Design review of the part shown in the three views and the two pictorial views. Dimensions are in mm from the part's minimum x, y and z. A direction names the side the tool comes from. Coordinates: 2 decimals unless noted, no trailing zeros. Order: outer loops, then holes, each group sorted by start corner. A loop starts at its lowest first (then second) coordinate and runs counter-clockwise, first axis right, second up. Notation, with made-up numbers: (66.5, 69.5) -> (83.5, 69.5) arc R17 ccw to (83.5, 84.5) -> close; hole circle Ø11 at (47.25, 12). An arc over 180 degrees is marked (long way). Answer as a JSON object with one key per item and string values. Group by question number.
1) Wall thickness on L1, parallel to Z at x = 47, y = 11.5; L2, parallel to X at y = 7, z = 19.5; L3, parallel to Y at x = 14, z = 3: over which ranges is each line inside the solid? List them lowest first.
2) Add section A-A, the plane x = 25. Write out the cut boundary in (y, z), then the cut area to 3 significant figures.
3) Add section B-B, the plane y = 6.5. Write out the cut boundary in (x, z), then the cut area to 3 significant figures.
4) Add section D-D, the plane x = 10. Write out the cut boundary in (y, z).
5) For pin 1 (1.6 mm diameter, centred on x = 25.5, z = 38.5, fed in from -Y); pin 2 (13 mm diameter, centred on x = 29, y = 5.5, fed in from +Z); pin 3 (12 mm diameter, centred on x = 16.5, y = 17, fed in from -Z), all flat-tipped, find the tip position at first contact; note any pin that passes through.
6) Add section C-C, the plane z = 33.5. Write out the cut boundary in (x, y).
7) Machinability: for the marked faces 1, 2 and 3, which of the approach directions +Z, -Z, +X, -X, +Y, -Y give a long, thin tool a straight path to every point of the face, cutting with its end or side? Answer none if there is none.
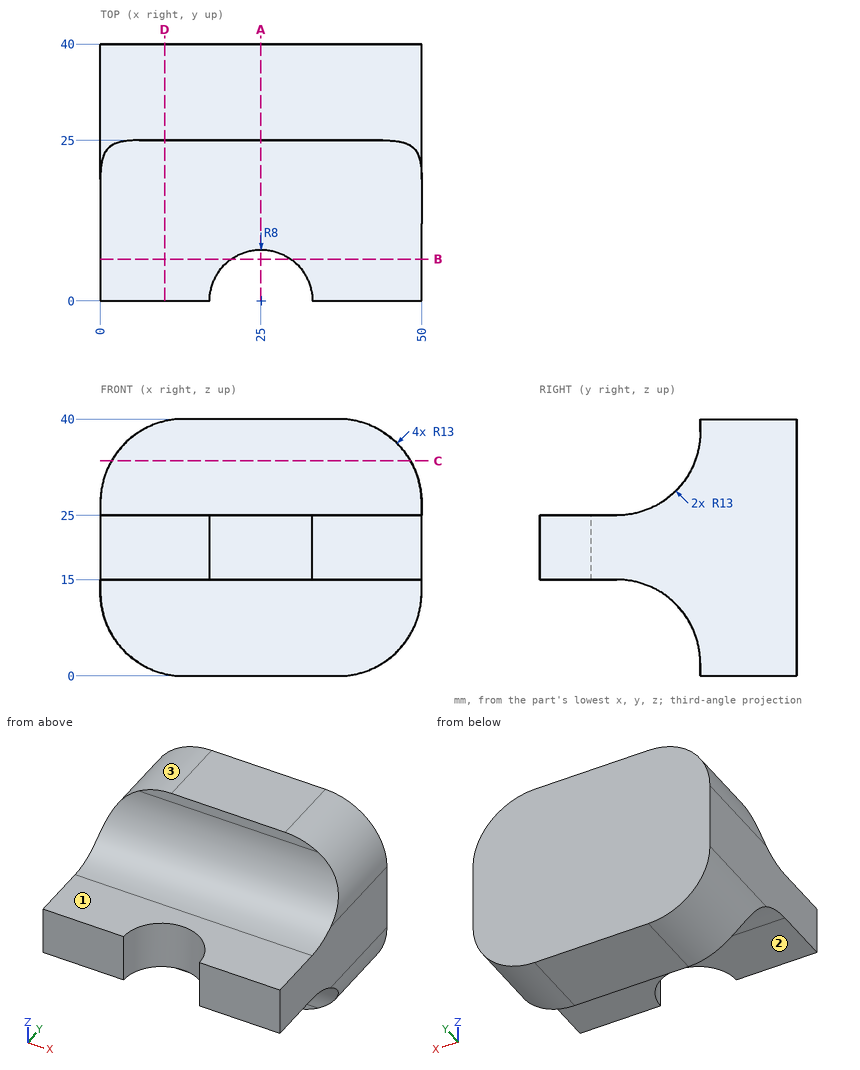
Output values:
{
 "1": {"L1": "z = 15 to 25", "L2": "x = 0 to 21.13, 28.87 to 50", "L3": "y = 24.96 to 40"},
 "2": {"outline": "(8, 15) -> (12, 15) arc R13 cw to (25, 2) -> (25, 0) -> (40, 0) -> (40, 40) -> (25, 40) -> (25, 38) arc R13 cw to (12, 25) -> (8, 25) -> close", "area": "843 mm²"},
 "3": {"outline": "(0, 15) -> (20.34, 15) -> (20.34, 25) -> (0, 25) -> close; (29.66, 15) -> (50, 15) -> (50, 25) -> (29.66, 25) -> close", "area": "407 mm²"},
 "4": {"outline": "(0, 15) -> (12, 15) arc R13 cw to (25, 2) -> (25, 0.35) -> (40, 0.35) -> (40, 39.65) -> (25, 39.65) -> (25, 38) arc R13 cw to (12, 25) -> (0, 25) -> close"},
 "5": {"pin 1": "stops at y = 25", "pin 2": "stops at z = 25", "pin 3": "stops at z = 8.93"},
 "6": {"outline": "(1.74, 24.2) -> (48.26, 24.2) -> (48.26, 40) -> (1.74, 40) -> close"},
 "7": {"face 1": "+Z, +X, -X, -Y", "face 2": "-Z, +X, -X, -Y", "face 3": "+Z, -X, +Y, -Y"}
}
